Autodesk Inventor part; units mm, degrees
ref_plane "YZ Plane" through (0, 0, 0) normal (1, 0, 0) x (0, 1, 0)
ref_plane "XZ Plane" through (0, 0, 0) normal (0, 1, 0) x (-1, 0, 0)
ref_plane "XY Plane" through (0, 0, 0) normal (0, 0, 1) x (1, 0, 0)
sketch "Esquisse1" plane through (0, 0, 0) normal (0, 1, 0) x (-1, 0, 0)
  circle A0 centre (-28.5, 0) radius 3.5
  circle A1 centre (28.5, 0) radius 3.5
  line L0 (-35.5, 10) -> (35.5, 10)
  line L1 (35.5, 10) -> (35.5, -10)
  line L2 (35.5, -10) -> (-35.5, -10)
  line L3 (-35.5, -10) -> (-35.5, 10)
  line L4 (-28.5, 0) -> (28.5, 0)
  point P0 (0, 0)
  dimension "d0" = 7
  dimension "d1" = 7
  dimension "d2" = 28.5
  dimension "d3" = 28.5
  dimension "d4" = 20
  dimension "d5" = 10
  dimension "d6" = 7
  dimension "d7" = 7
extrude "Extrusion1" add sketch "Esquisse1" along normal blind 22
sketch "Esquisse2" plane through (0, 22, 0) normal (0, 1, 0) x (1, 0, 0)
  circle A0 centre (-28.5, 0) radius 3.5
  circle A1 centre (28.5, 0) radius 3.5
  line L0 (-23.5, 7.5) -> (23.5, 7.5)
  line L1 (23.5, 7.5) -> (23.5, -7.5)
  line L2 (23.5, -7.5) -> (-23.5, -7.5)
  line L3 (-23.5, -7.5) -> (-23.5, 7.5)
  point P0 (0, 0)
  dimension "d10" = 15
  dimension "d11" = 7.5
  dimension "d12" = 5
  dimension "d13" = 5
extrude "Extrusion2" cut sketch "Esquisse2" against normal through all contours L0 L1 L2 L3
sketch "Esquisse3" plane through (-35.5, 0, 10) normal (0, 0, 1) x (1, 0, 0)
  line L0 (71, 0) -> (0, 0)
  line L1 (71, 0) -> (71, 22)
  line L2 (0, 22) -> (71, 22)
  line L3 (0, 0) -> (0, 22)
  line L4 (14, 22) -> (57, 22)
  line L5 (57, 22) -> (57, 0)
  line L6 (57, 0) -> (14, 0)
  line L7 (14, 0) -> (14, 22)
  line L8 (14, 22) -> (22, 22)
  line L9 (22, 22) -> (22, 14)
  line L10 (22, 14) -> (14, 14)
  line L11 (14, 14) -> (14, 22)
  line L12 (57, 22) -> (49, 22)
  line L13 (49, 22) -> (49, 14)
  line L14 (49, 14) -> (57, 14)
  line L15 (57, 14) -> (57, 22)
  line L16 (14, 22) -> (22, 14)
  line L17 (22, 22) -> (14, 14)
  line L18 (49, 14) -> (57, 22)
  line L19 (49, 22) -> (57, 14)
  circle A0 centre (18, 18) radius 2
  circle A1 centre (53, 18) radius 2
  point P0 (35.5, 0)
  dimension "d16" = 14
  dimension "d17" = 14
  dimension "d18" = 8
  dimension "d19" = 8
  dimension "d20" = 8
  dimension "d21" = 8
  dimension "d22" = 4
  dimension "d23" = 4
sketch "Esquisse4" plane through (35.5, 0, 10) normal (1, 0, 0) x (0, 0, -1)
  line L0 (20, 0) -> (0, 0)
  line L1 (0, 22) -> (20, 22)
  line L2 (7, 22) -> (13, 22)
  line L3 (13, 22) -> (13, 0)
  line L4 (13, 0) -> (7, 0)
  line L5 (7, 0) -> (7, 22)
  circle A0 centre (3.5, 7.5) radius 1.5
  circle A1 centre (16.5, 7.5) radius 1.5
  line L6 (20, 0) -> (20, 22)
  line L7 (0, 0) -> (7, 0)
  line L8 (7, 0) -> (7, 15)
  line L9 (7, 15) -> (0, 15)
  line L10 (0, 15) -> (0, 0)
  line L11 (13, 0) -> (20, 0)
  line L12 (20, 0) -> (20, 15)
  line L13 (20, 15) -> (13, 15)
  line L14 (13, 15) -> (13, 0)
  line L15 (0, 15) -> (7, 0)
  line L16 (7, 15) -> (0, 0)
  line L17 (13, 15) -> (20, 0)
  line L18 (20, 15) -> (13, 0)
  point P0 (10, 0)
  dimension "d26" = 6
  dimension "d27" = 3
  dimension "d28" = 3
  dimension "d29" = 3
  dimension "d32" = 15
extrude "Extrusion4" cut sketch "Esquisse4" against normal through all contours L17 L18 A1 | A1 L18 L17 | A1 L17 L18 | L18 L17 A1 | L15 L16 A0 | A0 L16 L15 | A0 L15 L16 | L16 L15 A0
sketch "Esquisse5" plane through (-35.5, 0, 10) normal (0, 0, 1) x (1, 0, 0)
  line L0 (71, 0) -> (0, 0)
  line L1 (71, 0) -> (71, 22)
  line L2 (0, 0) -> (71, 0)
  line L3 (71, 0) -> (71, 11)
  line L4 (71, 11) -> (0, 11)
  line L5 (0, 11) -> (0, 0)
  point P0 (35.5, 0)
  dimension "d33" = 11
extrude "Extrusion5" cut sketch "Esquisse5" against normal through all
sketch "Esquisse6" plane through (0, 22, 0) normal (0, 1, 0) x (1, 0, 0)
  line L0 (23.5, 7.5) -> (23.5, -7.5)
  line L1 (-35.5, -10) -> (35.5, -10)
  line L2 (-23.5, -7.5) -> (23.5, -7.5)
  line L3 (23.5, -7.5) -> (23.5, -10)
  line L4 (23.5, -10) -> (-23.5, -10)
  line L5 (-23.5, -10) -> (-23.5, -7.5)
  line L6 (-35.5, -10) -> (-23.5, -10)
  line L7 (-23.5, -10) -> (-23.5, -7.5)
  line L8 (-23.5, -7.5) -> (-35.5, -7.5)
  line L9 (-35.5, -7.5) -> (-35.5, -10)
  line L10 (35.5, -10) -> (23.5, -10)
  line L11 (23.5, -10) -> (23.5, -7.5)
  line L12 (23.5, -7.5) -> (35.5, -7.5)
  line L13 (35.5, -7.5) -> (35.5, -10)
  point P0 (0, 0)
extrude "Extrusion6" cut sketch "Esquisse6" against normal through all
extrude "Extrusion8" add sketch "Esquisse3" against normal through all contours A1 L18 L19 | L19 L18 A1 | L18 L19 A1 | A0 L16 L17 | L17 L16 A0 | A1 L19 L18 | A0 L17 L16 | L16 L17 A0
fillet "Congé1" radius 3 2 edges at (35.5, 16.5, -10) (-35.5, 16.5, -10)
equation "\"d5\" = 0.5 * d4"
equation "\"d17\" = d16"
properties part number "tendeur_base_up"
Verification items for the finished model (mm, model axes). A direction names the side the tool comes from. Round coordinates to 2 decimals unless told otherwise and drop trailing zeros. Write each loop counter-clockwise with the first axis right and the second up, starting at its lowest first coordinate (ties: lowest second). Pieces come first, ordered by that corner, then holes. Notation, with made-up numbers: (72, 33.25) -> (110, 33.25) arc R8 cw to (110, 46.25) -> close; hole circle Ø4 at (48, 11). An arc over 180 degrees is marked (long way). Write each question's results on one line, items separated by ' | '. Start each with the question number.
1. Set-up check for faces 5 (the cylindrical face through (17.24, 19.983, 1.373)), 6 (the flat face through (23.5, 17, 0)), 7 (the flat face through (-29, 17, 7.5)): record each of +Z, -Z, +X, -X, +Y, -Y from which the full face is reachable in a straight line by a thin tool's end or side.
2. Material ranges on probe 1 along X at (y, z) = (14.75, 0); probe 2 along Z at (x, y) = (28.5, 15.5); probe 3 along X at (y, z) = (16.25, 0), recorded low to high. Write a range as from..to.
3. Draft check along X on faces 1 (the flat face through (0, 17, -7.5)), 2 (the cylindrical face through (-17.76, 19.983, 1.373)), 3 (the flat face through (8, 11, -9)), 4 (the cylindrical face through (34.64, 16.58, -9.1)). Enter one of: +X half, -X half, draft (parallel to the pull), parting line (faces both ways), or undercut.
4. Cross-section at B-B (y = 18). Enter the section's corners in (x, z), then the cut area to 3 significant figures.
5. Cross-section at A-A (z = 0). Enter the section's corners in (x, y), then the cut area to 3 significant figures.
6. Depth check by flat-ended pin: P1, Ø3, axis at x = -15.5, z = -2, coming from the +Y side; P2, Ø2, axis at x = 19.5, y = 12.5, coming from the +Z side; P3, Ø4, axis at x = 28.5, z = 0, coming from the +Y side. Enter the tip coordinate at first touch or a pass-through.
7. Cross-section at D-D (x = -17.5). Enter the section's corners in (y, z), then the cut area to 3 significant figures.
8. Cross-section at C-C (x = -28.5). Enter the section's corners in (y, z).
Solutions:
1) face 5: +Z | face 6: +Z, +Y, -Y | face 7: +Z, -X, +Y, -Y
2) probe 1: x = -35.5..-32, -25..-23.5, 23.5..25, 32..35.5 | probe 2: z = -10..-3.5, 3.5..7.5 | probe 3: x = -35.5..-32, -25..-23.5, -18.47..-16.53, 16.53..18.47, 23.5..25, 32..35.5
3) face 1: undercut | face 2: undercut | face 3: draft | face 4: +X half
4) outline: (-35.5, -7) arc R3 ccw to (-32.5, -10) -> (-19.5, -10) -> (15.5, -10) -> (32.5, -10) arc R3 ccw to (35.5, -7) -> (35.5, 7.5) -> (23.5, 7.5) -> (23.5, -7.5) -> (19.5, -7.5) -> (19.5, 10) -> (15.5, 10) -> (15.5, -7.5) -> (-15.5, -7.5) -> (-15.5, 10) -> (-19.5, 10) -> (-19.5, -7.5) -> (-23.5, -7.5) -> (-23.5, 7.5) -> (-35.5, 7.5) -> close; hole circle Ø7 at (-28.5, 0); hole circle Ø7 at (28.5, 0) | area: 597 mm2
5) outline: (-35.5, 11) -> (-32, 11) -> (-32, 22) -> (-35.5, 22) -> close; (-25, 11) -> (-23.5, 11) -> (-23.5, 22) -> (-25, 22) -> close; circle Ø4 at (-17.5, 18); circle Ø4 at (17.5, 18); (23.5, 11) -> (25, 11) -> (25, 22) -> (23.5, 22) -> close; (32, 11) -> (35.5, 11) -> (35.5, 22) -> (32, 22) -> close | area: 135 mm2
6) P1: stops at y = 19.94 | P2: stops at z = -7.5 | P3: passes through
7) outline: (11, -10) -> (20, -10) -> (22, -10) -> (22, -7.5) -> (20, -7.5) -> (20, 10) -> (16, 10) -> (16, -7.5) -> (11, -7.5) -> close | area: 97.5 mm2
8) outline: (11, -10) -> (22, -10) -> (22, -3.5) -> (11, -3.5) -> close; (11, 3.5) -> (22, 3.5) -> (22, 7.5) -> (11, 7.5) -> close
